Work out the finished part from the listing and answer in its coordinate system (mm). A direction names the side the tool comes from. Round coordinates to 2 decimals unless told otherwise and drop trailing zeros. Loops run counter-clockwise (first coordinate to the right, second up) from the corner with the lowest first, then second, coordinate; pieces in that order, holes last.
from build123d import *

# Parameters (mm, degrees)
BOSS_EXTRUDE1_DEPTH      = 57.5
BOSS_EXTRUDE1_DEPTH_BACK = 42.5
BOSS_EXTRUDE2_DEPTH      = 67.5
BOSS_EXTRUDE2_DEPTH_BACK = 52.5
SKETCH2_W                = 20
SKETCH2_H                = 15
BOSS_EXTRUDE3_START      = 15
BOSS_EXTRUDE3_DEPTH      = 15
CUT_EXTRUDE1_DEPTH       = 106.901893724
CUT_EXTRUDE2_DEPTH       = 101.370563414
CUT_EXTRUDE2_DEPTH_BACK  = 101.370563414
SKETCH5_W                = 29
SKETCH5_H                = 40


with BuildPart() as part:
    # Sketch1 → Boss-Extrude1 (new, two sides: drawn at the far end of the back side and taken through both)
    with BuildSketch(Plane(origin=(0, 0, 0), x_dir=(0, 0, -1), z_dir=(1, 0, 0)).offset(-BOSS_EXTRUDE1_DEPTH_BACK)):
        with BuildLine():
            Line((0, -10), (-20, -10))
            Line((-20, -10), (-20, -25))
            Line((-20, -25), (20, -25))
            Line((20, -25), (20, -49.081564767))
            ThreePointArc((20, -49.081564767), (52.742771868, 5.215363425), (10, 52.048054719))
            Line((10, 52.048054719), (10, 0))
            ThreePointArc((10, 0), (7.071067812, -7.071067812), (0, -10))
        make_face()
    extrude(amount=BOSS_EXTRUDE1_DEPTH + BOSS_EXTRUDE1_DEPTH_BACK)

    # Sketch2 → Boss-Extrude2 (add, two sides: drawn at the far end of the back side and taken through both)
    with BuildSketch(Plane(origin=(0, 0, 0), x_dir=(0, 0, -1), z_dir=(1, 0, 0)).offset(-BOSS_EXTRUDE2_DEPTH_BACK)):
        with Locations((15, 29.548054719)):
            Rectangle(SKETCH2_W, SKETCH2_H)
    extrude(amount=BOSS_EXTRUDE2_DEPTH + BOSS_EXTRUDE2_DEPTH_BACK)

    # Sketch3 → Boss-Extrude3 (add)
    with BuildSketch(Plane.ZY.offset(42.5).offset(BOSS_EXTRUDE3_START)):
        with BuildLine():
            Line((20, -25), (-20, -25))
            Line((-20, -25), (-20, -49.081564767))
            ThreePointArc((-20, -49.081564767), (-42.679392836, -31.424026273), (-52.80652364, -4.524495668))
            Line((-52.80652364, -4.524495668), (20, -20))
            Line((20, -20), (20, -25))
        make_face()
    extrude(amount=-BOSS_EXTRUDE3_DEPTH)

    # Sketch4 → Cut-Extrude1 (cut, through all)
    with BuildSketch(Plane(origin=(0, -10, 0), x_dir=(1, 0, 0), z_dir=(0, 1, 0))):
        with BuildLine():
            Line((-32.5, -5), (47.5, -5))
            ThreePointArc((47.5, -5), (52.5, -10), (47.5, -15))
            Line((47.5, -15), (-32.5, -15))
            ThreePointArc((-32.5, -15), (-37.5, -10), (-32.5, -5))
        make_face()
    extrude(amount=-CUT_EXTRUDE1_DEPTH, mode=Mode.SUBTRACT)

    # Sketch5 → Cut-Extrude2 (cut, two sides: drawn at the far end of the back side and taken through both)
    with BuildSketch(Plane.XY.offset(-CUT_EXTRUDE2_DEPTH_BACK)):
        with Locations((2, 32.048054719)):
            Rectangle(SKETCH5_W, SKETCH5_H)
    extrude(amount=CUT_EXTRUDE2_DEPTH + CUT_EXTRUDE2_DEPTH_BACK, mode=Mode.SUBTRACT)


solid = part.part
Item 1: Section B-B, the plane x = -28 is taken. Give the vertices of the cut face in (y, z), plus the area to 3 significant figures.
Item 2: Straight lines are drawn through the part: line 1 (Y direction, x = 33.5, z = 16); line 2 (Z direction, x = -49, y = 34.5); line 3 (X direction, y = -5.5, z = -37.5). For each, find the intervals that lie inside material, in ascending order.
Item 3: Section C-C, the plane z = 10 is taken. Give the vertices of the cut face in (x, y), plus the area to 3 significant figures.
Item 4: Section D-D, the plane y = 30.5 is taken. Give the vertices of the cut face in (x, z).
Item 5: Each of these flat-tipped pins is pushed along its axis until it touches: P1, Ø10, axis at x = 20.5, y = 15, coming from the +Z side; P2, Ø10, axis at x = 35.5, z = -11, coming from the -Y side; P3, Ø4.5, axis at x = -36.5, y = 31.5, coming from the +Z side; P4, Ø22, axis at x = -29, z = -17.5, coming from the +Y side. Where does it stop, or does it pass through?
Item 6: Section A-A, the plane x = -9 is taken. Give the vertices of the cut face in (y, z).
Item 7: Determine the mould class of faces 1 (the face through (52.5, -17.4, 9.9)), 2 (the face through (42, 29, -5)), 3 (the face through (-57.5, -22, -24)) for opening direction X: pulls with the +X half, pulls with the -X half, needs draft (parallel to the pull), parting line crosses it, or undercut.
Item 8: For faces 4 (the face through (7, 11, -10)), 5 (the face through (-28, 45, -10)), 6 (the face through (16.5, 27, -23)), 7 (the face through (-42, 37.048, -8)), 8 (the face through (-42, 22.048, -8)), determine the directions among +Z, -Z, +X, -X, +Y, -Y from which every point of the face is accessible in a straight line to the end or side of a thin tool.
Answer below:
1. outline: (-49.08, -20) arc R53 ccw to (52.05, -10) - (37.05, -10) - (37.05, -5) - (22.05, -5) - (22.05, -10) - (0, -10) arc R10 cw to (-10, 0) - (-10, 5) - (-25, 5) - (-25, -20) - close; (-25, 15) - (-10, 15) - (-10, 20) - (-25, 20) - close
1. area: 3,500 mm2
2. line 1: y = -25 to -10
2. line 2: z = -25 to -5
2. line 3: x = -42.5 to 57.5
3. outline: (-57.5, -25) - (-37.5, -25) - (-37.5, -10) - (-42.5, -10) - (-42.5, -17.87) - (-57.5, -17.87) - close; (52.5, -25) - (57.5, -25) - (57.5, -10) - (52.5, -10) - close
3. area: 257 mm2
4. outline: (-52.5, -25) - (-42.5, -25) - (-42.5, -43.34) - (-12.5, -43.34) - (-12.5, -5) - (-52.5, -5) - close; (16.5, -43.34) - (57.5, -43.34) - (57.5, -25) - (67.5, -25) - (67.5, -5) - (16.5, -5) - close
5. P1: stops at z = -10
5. P2: stops at y = -25
5. P3: stops at z = -5
5. P4: stops at y = 52.05
6. outline: (-49.08, -20) arc R53 ccw to (12.05, -51.61) - (12.05, -10) - (0, -10) arc R10 cw to (-10, 0) - (-10, 5) - (-25, 5) - (-25, -20) - close; (-25, 15) - (-10, 15) - (-10, 20) - (-25, 20) - close
7. face 1: undercut
7. face 2: needs draft
7. face 3: pulls with the -X half
8. face 4: +Z, +X, -X
8. face 5: +Z, +X, -X, +Y
8. face 6: +Z, -Z, +Y
8. face 7: +Z, -X, +Y
8. face 8: +Z, -X
